Check sheet for the modelled part. Datum: model origin and axes. Units: mm. Face numbers are marked on the shaded views. A direction names the side the tool comes from. Coordinates: 2 decimals unless noted, no trailing zeros. Write each loop counter-clockwise with the first axis right and the second up, starting at its lowest first coordinate (ties: lowest second). Pieces come first, ordered by that corner, then holes. Notation, with made-up numbers: M 26.25,67 L 33.25,67 A31 cw 33.25,104 Z; hole C 32,88 d3. An arc over 180 degrees is marked long. Answer as CSV lines item,"result". Start each with the question number.
1) Go/stop test with flat-tipped pins: pin 1 Ø8 at (x, z) = (57.15, -19.05) entering from +Y; pin 2 Ø6.5 at (x, y) = (279.4, 15.875) entering from +Z; pin 3 Ø9.5 at (x, y) = (126.5, 13.5) entering from -Z (3 decimals); pin 4 Ø2 at (x, z) = (99.5, -3.5) entering from -Y. Record where each tip stops, or that it passes through.
2) Access from +Z, -Z, +X, -X, +Y, -Y to the whole of each face (thin tool, end or side, straight path). Record for the marked faces 1 and 2.
3) Section check A-A (x = 233). Record the cut outline in (y, z) (3 decimals), and give its area (3 significant figures).
4) Material ranges on L1, parallel to X at y = -2.35, z = -19.05; L2, parallel to Z at x = 156.5, y = 19.75 (3 decimals), recorded low to high. Write a range as [from, to].
from build123d import *

# Parameters (mm, degrees)
SKETCH9_W                    = 323.85
SKETCH9_H                    = 28.575
BASE_FLANGE2_DEPTH           = 3.175
EDGE_FLANGE1_STRIP_W         = 19.05
EDGE_FLANGE1_STRIP_H         = 3.175
EDGE_FLANGE1_STRIP_CUT_DEPTH = 323.85
EDGE_FLANGE1_DEPTH           = 323.85
SKETCH15_R                   = 2.4511
CUT_EXTRUDE1_DEPTH           = 3.175
FILLET1_R                    = 3.175
SKETCH16_R                   = 2.4511
CUT_EXTRUDE2_DEPTH           = 3.175


# Sheet-metal steps are written as plain solids
with BuildPart() as part:
    # Sketch9 → Base-Flange2 (new body)
    with BuildSketch(Plane(origin=(0, 0, 0), x_dir=(1, 0, 0), z_dir=(0, 1, 0))):
        with Locations((161.925, 14.2875)):
            Rectangle(SKETCH9_W, SKETCH9_H)
    extrude(amount=-BASE_FLANGE2_DEPTH)

    # Edge-Flange1 strip (across the edge) → Edge-Flange1 strip cut (cut)
    with BuildSketch(Plane(origin=(0, 0, 0), x_dir=(0, 0, -1), z_dir=(1, 0, 0))):
        with Locations((-3.175, -1.5875)):
            Rectangle(EDGE_FLANGE1_STRIP_W, EDGE_FLANGE1_STRIP_H)
    extrude(amount=EDGE_FLANGE1_STRIP_CUT_DEPTH, mode=Mode.SUBTRACT)

    # Edge-Flange1 section (across the edge) → Edge-Flange1 (add)
    with BuildSketch(Plane(origin=(0, 0, 0), x_dir=(0, 0, -1), z_dir=(1, 0, 0))):
        with BuildLine():
            Line((0, 3.175), (0, 22.225))
            Line((0, 22.225), (3.175, 22.225))
            Line((3.175, 22.225), (3.175, 3.175))
            ThreePointArc((3.175, 3.175), (4.10493597, 0.92993597), (6.35, 0))
            Line((6.35, 0), (6.35, -3.175))
            ThreePointArc((6.35, -3.175), (1.859871939, -1.315128061), (0, 3.175))
        make_face()
    extrude(amount=EDGE_FLANGE1_DEPTH)

    # Sketch15 → Cut-Extrude1 (cut)
    with BuildSketch(Plane(origin=(0, 0, 0), x_dir=(1, 0, 0), z_dir=(0, 1, 0))):
        with Locations(Location((19.05, 19.05, 0), (0, 0, 270))):
            Circle(SKETCH15_R)
        with Locations(Location((57.15, 19.05, 0), (0, 0, 270))):
            Circle(SKETCH15_R)
        with Locations(Location((279.4, 19.05, 0), (0, 0, 270))):
            Circle(SKETCH15_R)
        with Locations((501.65, 19.05)):
            Circle(SKETCH15_R)
    extrude(amount=-CUT_EXTRUDE1_DEPTH, mode=Mode.SUBTRACT)

    # Fillet1
    fillet1_edges = [part.edges().sort_by_distance(p)[0] for p in [
        (0, 22.225, -1.5875),
        (323.85, 22.225, -1.5875),
        (0, -1.5875, -28.575),
        (323.85, -1.5875, -28.575),
    ]]
    fillet(fillet1_edges, radius=FILLET1_R)

    # Sketch16 → Cut-Extrude2 (cut)
    with BuildSketch(Plane.XY):
        with Locations((19.05, 15.875)):
            Circle(SKETCH16_R)
        with Locations((57.15, 15.875)):
            Circle(SKETCH16_R)
        with Locations((279.4, 15.875)):
            Circle(SKETCH16_R)
    extrude(amount=-CUT_EXTRUDE2_DEPTH, mode=Mode.SUBTRACT)


solid = part.part
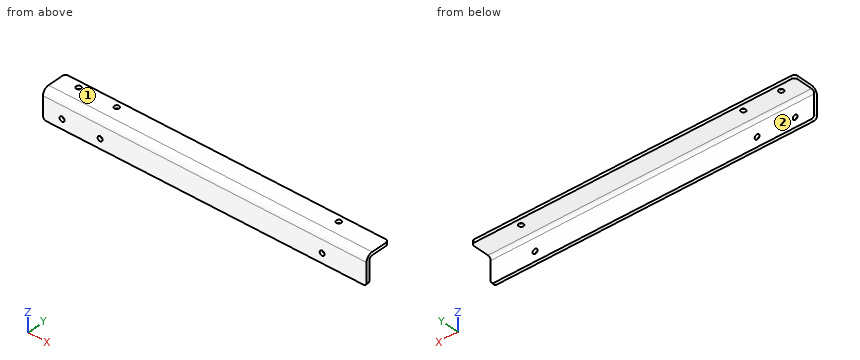
Results found:
1,pin 1,"stops at y = 0"
1,pin 2,"stops at z = 0"
1,pin 3,"stops at z = -3.175"
1,pin 4,"stops at y = -2.9"
2,face 1,"+Z, +X, -X, +Y, -Y"
2,face 2,"-Z, +X, -X, +Y"
3,outline,"M -3.175,-28.575 L 0,-28.575 L 0,-6.35 A3.175 cw 3.175,-3.175 L 22.225,-3.175 L 22.225,0 L 3.175,0 A6.35 ccw -3.175,-6.35 Z"
3,area,"155 mm2"
4,L1,"x = [0, 16.6], [21.5, 54.7], [59.6, 276.95], [281.85, 323.85]"
4,L2,"z = [-3.175, 0]"
